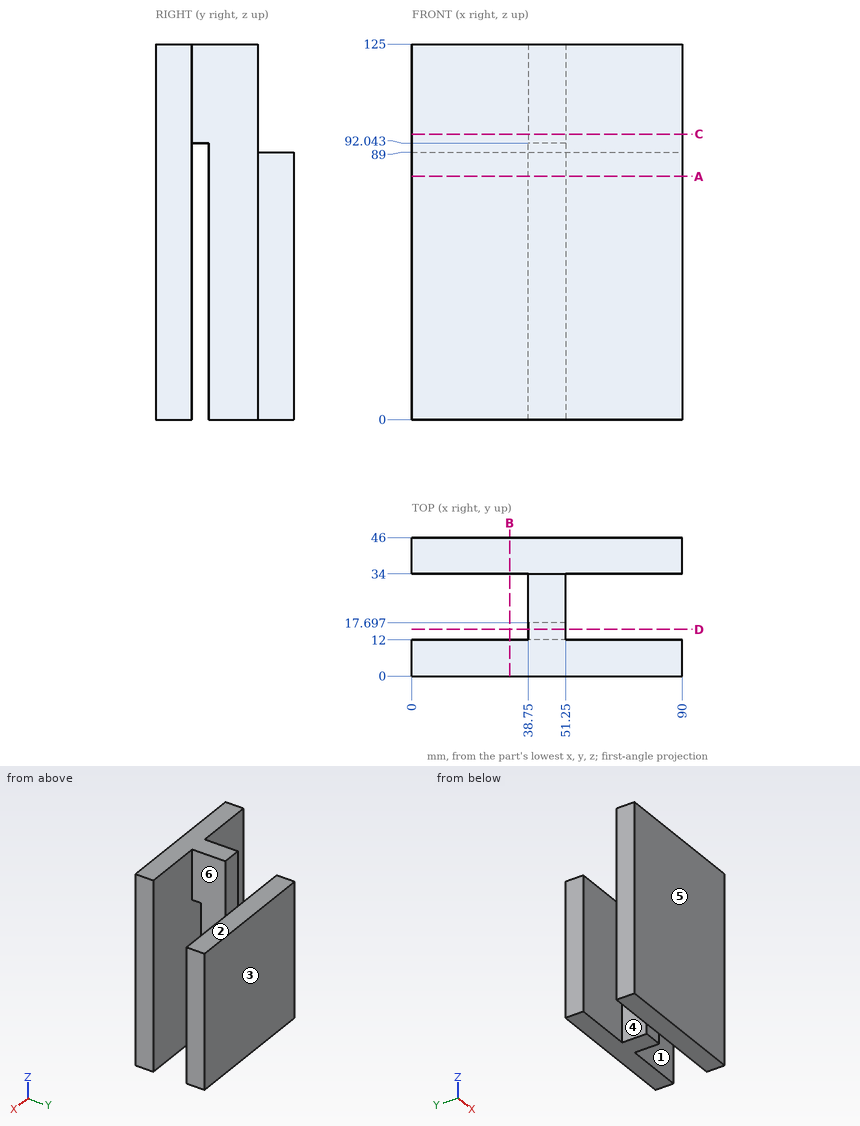
Design review of the part shown in the three views and the two pictorial views. Dimensions are in mm from the part's minimum x, y and z. A direction names the side the tool comes from. Coordinates: 2 decimals unless noted, no trailing zeros. Loops run counter-clockwise (first coordinate to the right, second up) from the corner with the lowest first, then second, coordinate; pieces in that order, holes last.
(1) Consider section A-A, the plane z = 81. Give the boundary of the cut face in (x, y).
Determined:
outline: (0, 0) - (90, 0) - (90, 12) - (0, 12) - close; (0, 34) - (38.75, 34) - (38.75, 17.7) - (51.25, 17.7) - (51.25, 34) - (90, 34) - (90, 46) - (0, 46) - close
(2) Consider section D-D, the plane y = 15.5. Give the boundary of the cut face in (x, z).
Determined:
outline: (38.75, 92.04) - (51.25, 92.04) - (51.25, 125) - (38.75, 125) - close
(3) Consider section B-B, the plane x = 32.5. Give the boundary of the cut face in (y, z), plus the area to 3 significant figures.
Determined:
outline: (0, 0) - (12, 0) - (12, 125) - (0, 125) - close; (34, 0) - (46, 0) - (46, 89) - (34, 89) - close
area: 2,570 mm2
(4) Tool access review of the marked faces 4, 5 and 6: name each direction out of +Z, -Z, +X, -X, +Y, -Y from which nothing blocks a thin tool from reaching the whole face with its end or side.
Determined:
face 4: +Z, -Z, -X
face 5: +Z, -Z, +X, -X, -Y
face 6: +Z, -Z, +X
(5) Insertion check: P1, Ø6, axis at x = 47.5, z = 26, coming from the -Y side; P2, Ø3.5, axis at x = 35.5, y = 39, coming from the +Z side; P3, Ø1.7, axis at x = 46, y = 16, coming from the -Z side; P4, Ø14, axis at x = 45.5, z = 102, coming from the +Y side. Each pin has a flat end and moves straight along its axis. Give the tip position at first contact, or say it passes through.
Determined:
P1: stops at y = 0
P2: stops at z = 89
P3: stops at z = 92.04
P4: stops at y = 34
(6) Draft analysis for pull direction Y (two halves, no side actions). For the marked faces 1, 2 and 3, state which applies: +Y half, -Y half, draft (parallel to the pull), parting line (faces both ways), or undercut.
Determined:
face 1: undercut
face 2: draft
face 3: +Y half
(7) Consider section C-C, the plane z = 95. Give the boundary of the cut face in (x, y), plus the area to 4 significant figures.
Determined:
outline: (0, 0) - (90, 0) - (90, 12) - (51.25, 12) - (51.25, 34) - (38.75, 34) - (38.75, 12) - (0, 12) - close
area: 1,355 mm2
(8) Wall thickness on L1, parallel to Y at x = 48, z = 43; L2, parallel to Y at x = 32.5, z = 66; L3, parallel to Y at x = 45, z = 111: over which ranges is each line inside the solid? List them lowest first.
Determined:
L1: y = 0 to 12, 17.7 to 46
L2: y = 0 to 12, 34 to 46
L3: y = 0 to 34
